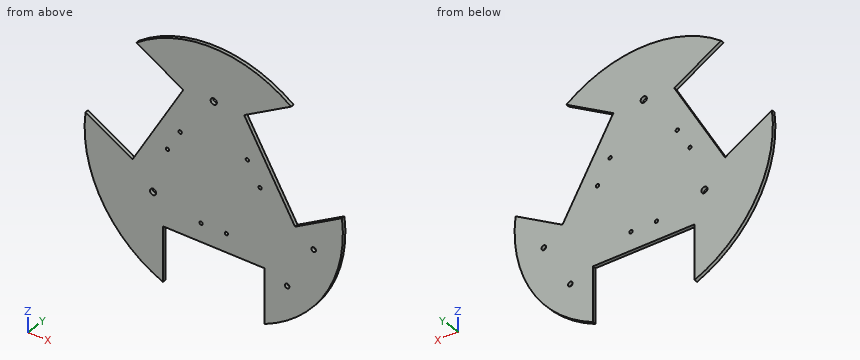
from build123d import *

# Parameters (mm, degrees)
SKETCH1_R           = 2.1463
SKETCH1_R_2         = 1.14935
SKETCH1_R_3         = 1.5875
BOSS_EXTRUDE1_DEPTH = 2.3622


with BuildPart() as part:
    # Sketch1 → Boss-Extrude1 (new body)
    with BuildSketch(Plane(origin=(0, 0, 0), x_dir=(1, 0, 0), z_dir=(0, 1, 0))):
        with BuildLine():
            Line((-35, 44.411902139), (-35, 81.720315712))
            ThreePointArc((-35, 81.720315712), (-76.989658396, 44.45), (-88.271869412, -10.549268723))
            Line((-88.271869412, -10.549268723), (-55.961835482, 8.104938063))
            Line((-55.961835482, 8.104938063), (-20.961835482, -52.516840202))
            Line((-20.961835482, -52.516840202), (-53.271869412, -71.171046988))
            ThreePointArc((-53.271869412, -71.171046988), (0, -88.9), (53.271869412, -71.171046988))
            Line((53.271869412, -71.171046988), (20.961835482, -52.516840202))
            Line((20.961835482, -52.516840202), (55.961835482, 8.104938063))
            Line((55.961835482, 8.104938063), (88.271869412, -10.549268723))
            ThreePointArc((88.271869412, -10.549268723), (76.989658396, 44.45), (35, 81.720315712))
            Line((35, 81.720315712), (35, 44.411902139))
            Line((35, 44.411902139), (-35, 44.411902139))
        make_face()
        with Locations(Location((-41.747414599, 24.102881057, 0), (0, 0, 270))):
            Circle(SKETCH1_R, mode=Mode.SUBTRACT)
        with Locations(Location((-8.73125, 31.75, 0), (0, 0, 270))):
            Circle(SKETCH1_R_2, mode=Mode.SUBTRACT)
        with Locations(Location((50.529406911, 49.981355026, 0), (0, 0, 270))):
            Circle(SKETCH1_R_3, mode=Mode.SUBTRACT)
        with Locations(Location((0, -53.205762114, 0), (0, 0, 90))):
            Circle(SKETCH1_R, mode=Mode.SUBTRACT)
        with Locations(Location((68.785656911, 18.36060247, 0), (0, 0, 270))):
            Circle(SKETCH1_R_3, mode=Mode.SUBTRACT)
        with Locations(Location((8.73125, 31.75, 0), (0, 0, 270))):
            Circle(SKETCH1_R_2, mode=Mode.SUBTRACT)
        with Locations(Location((31.86193157, -8.313515693, 0), (0, 0, 270))):
            Circle(SKETCH1_R_2, mode=Mode.SUBTRACT)
        with Locations(Location((23.13068157, -23.436484307, 0), (0, 0, 270))):
            Circle(SKETCH1_R_2, mode=Mode.SUBTRACT)
        with Locations(Location((-31.86193157, -8.313515693, 0), (0, 0, 270))):
            Circle(SKETCH1_R_2, mode=Mode.SUBTRACT)
        with Locations(Location((-23.13068157, -23.436484307, 0), (0, 0, 270))):
            Circle(SKETCH1_R_2, mode=Mode.SUBTRACT)
    extrude(amount=BOSS_EXTRUDE1_DEPTH)


solid = part.part
Verification items for the finished model (mm, model axes). Coordinates: 2 decimals unless noted, no trailing zeros. Order: outer loops, then holes, each group sorted by start corner. A loop starts at its lowest first (then second) coordinate and runs counter-clockwise, first axis right, second up. Notation, with made-up numbers: M 31.25,79 L 63.25,79 A18 cw 63.25,95 Z; hole C 44,39.5 d9. An arc over 180 degrees is marked long. One line per item, written item: value. Start each with the question number.
Item 1: Sectioned sample at B-B on z = 0.5. Record the cut outline in (x, y).
Item 2: Depth check by flat-ended pin: P1, Ø4, axis at x = 50.53, z = -49.98, coming from the +Y side; P2, Ø1.4, axis at x = -8.73, z = -31.75, coming from the +Y side. Enter the tip coordinate at first touch or a pass-through.
Item 3: Sectioned sample at C-C on y = 1.35. Give the number of separate pieces and of enclosed holes in the cut face, then the cut area to 3 significant figures.
Item 4: Thickness scan on probe 1 along Z at (x, y) = (31, 1.7); probe 2 along X at (y, z) = (1.7, -19.5) (3 decimals); probe 3 along Z at (x, y) = (-50.5, 1.75). Record the ranges inside material, lowest first.
Item 5: Sectioned sample at A-A on x = 0. Record the cut outline in (y, z), then the cut area to 3 significant figures.
Calculated:
1. outline: M -88.9,0 L -70.87,0 L -70.87,2.36 L -88.9,2.36 Z; M -50.99,0 L 50.99,0 L 50.99,2.36 L -50.99,2.36 Z; M 70.87,0 L 88.9,0 L 88.9,2.36 L 70.87,2.36 Z
2. P1: y = 2.36
2. P2: through
3. separate pieces: 1
3. enclosed holes: 10
3. area: 15,900 mm^2
4. probe 1: -44.41 to 7.55, 9.07 to 35.13, 58.31 to 83.32
4. probe 2: -86.735 to 67.68, 69.891 to 86.735
4. probe 3: -73.16 to 1.36, 69.57 to 73.16
5. outline: M 0,-44.41 L 2.36,-44.41 L 2.36,51.06 L 0,51.06 Z; M 0,55.35 L 2.36,55.35 L 2.36,88.9 L 0,88.9 Z
5. area: 305 mm^2
